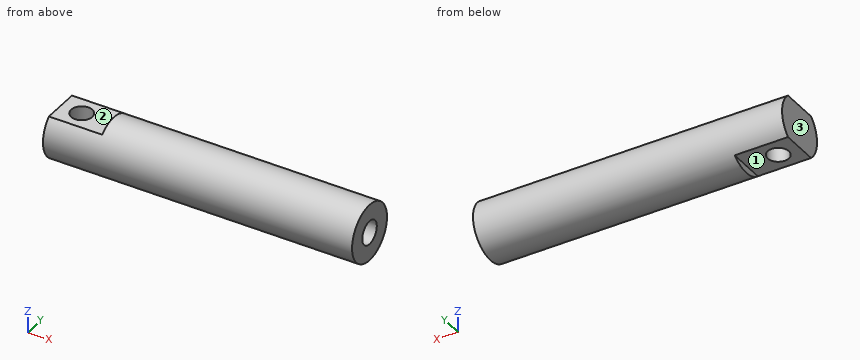
Autodesk Inventor part; units mm, degrees
ref_plane "Work Plane2" through (0, 0, -6) normal (0, 0, 1) x (-1, 0, 0)
ref_plane "YZ Plane" through (0, 0, 0) normal (1, 0, 0) x (0, 1, 0)
ref_plane "XZ Plane" through (0, 0, 0) normal (0, 1, 0) x (-1, 0, 0)
sketch "Sketch1" plane through (0, 0, 0) normal (1, 0, 0) x (0, 1, 0)
  circle A0 centre (0, 0) radius 8
  dimension "d0" = 16
extrude "Extrusion1" add sketch "Sketch1" against normal blind 87
ref_plane "Work Plane1" through (0, 0, 0) normal (0, 0, 1) x (-1, 0, 0)
sketch "Sketch2" plane through (0, 0, 0) normal (0, 0, 1) x (1, 0, 0)
  point P0 (0, 0)
ref_plane "Work Plane2" through (0, 0, -6) normal (0, 0, 1) x (-1, 0, 0)
sketch "Sketch3" plane through (0, 0, -6) normal (0, 0, 1) x (-1, 0, 0)
  line L0 (72, -14.6866) -> (87, -14.6866)
  line L1 (87, -14.6866) -> (87, 13.5616)
  line L2 (87, 13.5616) -> (72, 13.5616)
  line L3 (72, 13.5616) -> (72, -14.6866)
  line L4 (87, -8) -> (87, 8)
  point P0 (0, 0)
  dimension "d5" = 15
  dimension "d6" = 0
extrude "Extrusion2" cut sketch "Sketch3" against normal blind 87
mirror "Mirror1" about plane through (0, 0, 0) normal (0, 0, 1) of "Extrusion2"
sketch "Sketch4" plane through (0, 0, 0) normal (0, 0, 1) x (-1, 0, 0)
  circle A0 centre (81, 0) radius 3
  line L0 (87, -5.2915) -> (87, 5.2915)
  point P0 (0, 0)
  dimension "d9" = 6
  dimension "d10" = 6
extrude "Extrusion3" cut sketch "Sketch4" along normal mid plane 20
hole "Hole1" at (0, 0, 0) direction (-1, 0, 0) diameter 6.647 depth 50 tip angle 118
properties material "Steel"
Source: CAD feature listing. Evaluate the final solid. Frame: model axes, mm. Face numbers are marked on the shaded views. A direction names the side the tool comes from. Coordinates: 2 decimals unless noted, no trailing zeros. Loops run counter-clockwise (first coordinate to the right, second up) from the corner with the lowest first, then second, coordinate; pieces in that order, holes last. Notation, with made-up numbers: (-21, 21.25) -> (1, 21.25) arc R20 cw to (1, 26.25) -> close; hole circle Ø8 at (71.5, 45). An arc over 180 degrees is marked (long way). Answer in a Markdown table with one row per item. Add a question column.
Q1. Section C-C on x = -5.5. Return the cut outline in (y, z).
Q2. Section B-B on z = 4.5. Return the cut outline in (x, y), and give its area (3 significant figures).
Q3. Section A-A on x = -81. Return the cut outline in (y, z), and give its area (3 significant figures).
Q4. Reachability of the marked faces 1, 2 and 3 from +Z, -Z, +X, -X, +Y, -Y: full face, straight path, thin tool, end or side. Return the list, or none.
Q5. Ray query, line 1 along Y through (x, z) = (-15.5, 0); line 2 along Z through (x, y) = (-46.5, -6). Return the intervals inside material, ascending.
Q6. Contact query for flat-ended pins moving along their axis: pin 1 Ø1 at (x, y) = (-17.5, 3.5) entering from -Z; pin 2 Ø3 at (x, y) = (-37, -1.5) entering from -Z; pin 3 Ø8 at (x, y) = (-36.5, -5) entering from +Z; pin 4 Ø1.6 at (y, z) = (0.5, -7) entering from -X. Output: stop coordinate, or through.
Q7. Section D-D on y = 6.25. Return the cut outline in (x, z).
Computed values:
| question | item | result |
|---|---|---|
| 1 | outline | circle Ø16 at (0, 0); hole circle Ø6.65 at (0, 0) |
| 2 | outline | (-87, -6.61) -> (0, -6.61) -> (0, 6.61) -> (-87, 6.61) -> close; hole circle Ø6 at (-81, 0) |
| 2 | area | 1,120 mm^2 |
| 3 | outline | (-5.29, -6) -> (-3, -6) -> (-3, 6) -> (-5.29, 6) arc R8 ccw to start; (3, -6) -> (5.29, -6) arc R8 ccw to (5.29, 6) -> (3, 6) -> close |
| 3 | area | 100 mm^2 |
| 4 | face 1 | -Z, -X, +Y, -Y |
| 4 | face 2 | +Z, -X, +Y, -Y |
| 4 | face 3 | +Z, -Z, -X, +Y, -Y |
| 5 | line 1 | y = -8 to -3.32, 3.32 to 8 |
| 5 | line 2 | z = -5.29 to 5.29 |
| 6 | pin 1 | stops at z = -7.42 |
| 6 | pin 2 | stops at z = -8 |
| 6 | pin 3 | stops at z = 7.94 |
| 6 | pin 4 | stops at x = -72 |
| 7 | outline | (-87, -4.99) -> (0, -4.99) -> (0, 4.99) -> (-87, 4.99) -> close |
